```python
from build123d import *

# Parameters (mm, degrees)
BOSS_EXTRUDE1_DEPTH = 3


with BuildPart() as part:
    # Sketch2 → Boss-Extrude1 (new body)
    with BuildSketch(Plane.XY):
        with BuildLine():
            Line((-3.781717443, 11.388529895), (-2.521144962, 7.592353264))
            ThreePointArc((-2.521144962, 7.592353264), (-1.768998185, 7.801964203), (-1, 7.937253933))
            Line((-1, 7.937253933), (-1, 8.94427191))
            Line((-1, 8.94427191), (-1, 9.949874371))
            Line((-1, 9.949874371), (1, 9.949874371))
            Line((1, 9.949874371), (1, 8.94427191))
            Line((1, 8.94427191), (1, 7.937253933))
            ThreePointArc((1, 7.937253933), (8, 0), (1, -7.937253933))
            Line((1, -7.937253933), (1, -8.94427191))
            Line((1, -8.94427191), (1, -10.050125629))
            Line((1, -10.050125629), (-1, -10.050125629))
            Line((-1, -10.050125629), (-1, -8.94427191))
            Line((-1, -8.94427191), (-1, -7.937253933))
            ThreePointArc((-1, -7.937253933), (-1.768998185, -7.801964203), (-2.521144962, -7.592353264))
            Line((-2.521144962, -7.592353264), (-3.781717443, -11.388529895))
            ThreePointArc((-3.781717443, -11.388529895), (12, 0), (-3.781717443, 11.388529895))
        make_face()
    extrude(amount=BOSS_EXTRUDE1_DEPTH)


solid = part.part
```
Geometry: final body of the model. Coordinates: model frame, mm. A direction names the side the tool comes from. Round coordinates to 2 decimals unless told otherwise and drop trailing zeros. Write each loop counter-clockwise with the first axis right and the second up, starting at its lowest first coordinate (ties: lowest second). Pieces come first, ordered by that corner, then holes. Notation, with made-up numbers: (73, -25) -> (105, -25) arc R18 ccw to (105, -11) -> close; hole circle Ø3 at (43, -15). An arc over 180 degrees is marked (long way). Use CSV: the item, a comma, the result in double quotes. Start each with the question number.
Q1. Section B-B (z = 0.3). Return loops of the section in (x, y), plus the area to 3 significant figures.
Q2. Section A-A (x = 0). Return loops of the section in (y, z), plus the area to 3 significant figures.
Q3. First-contact query: pin 1 Ø0.6 at (x, z) = (-0.5, 1) entering from +Y; pin 2 Ø1.7 at (y, z) = (-8.5, 2) entering from -X; pin 3 Ø1.6 at (y, z) = (8.5, 2) entering from +X; pin 4 Ø8 at (x, y) = (-0.5, -1.5) entering from +Z. Flat tips, straight axial feed; report the tip coordinate or a pass-through.
Q4. Pull-direction query (X, two-part tool) for faces 4 (the face through (8, 3, 0)), 5 (the face through (1, -9, 1)), 6 (the face through (-3.16, 9.52, 1.48)); classes: pulls with the +X half, pulls with the -X half, needs draft (parallel to the pull), parting line crosses it, or undercut.
Q5. Section C-C (y = 0). Return loops of the section in (x, z).
Q6. Reachability of faces 1 (the face through (-3.14, -9.46, 1.48)), 2 (the face through (8, 3, 3)), 3 (the face through (8, 0, 1)) from +Z, -Z, +X, -X, +Y, -Y: full face, straight path, thin tool, end or side. Return the list, or none.
Q7. Line query: L1, parallel to Y at x = 0.5, z = 1.15; L2, parallel to Y at x = 3, z = 2.85; L3, parallel to X at y = 8, z = 0.35. Output: solid intervals per line, ascending.
Q8. Section D-D (x = 4.5). Return loops of the section in (y, z), plus the area to 3 significant figures.
Result sheet:
1,outline,"(-3.78, -11.39) arc R12 ccw (long way) to (-3.78, 11.39) -> (-2.52, 7.59) arc R8 cw to (-1, 7.94) -> (-1, 9.95) -> (1, 9.95) -> (1, 7.94) arc R8 cw to (1, -7.94) -> (1, -10.05) -> (-1, -10.05) -> (-1, -7.94) arc R8 cw to (-2.52, -7.59) -> close"
1,area,"143 mm²"
2,outline,"(-12, 0) -> (-10.05, 0) -> (-10.05, 3) -> (-12, 3) -> close; (9.95, 0) -> (12, 0) -> (12, 3) -> (9.95, 3) -> close"
2,area,"12.0 mm²"
3,pin 1,"y = 12"
3,pin 2,"x = -3.1"
3,pin 3,"x = 9.2"
3,pin 4,"through"
4,face 4,"needs draft"
4,face 5,"undercut"
4,face 6,"pulls with the -X half"
5,outline,"(8, 0) -> (12, 0) -> (12, 3) -> (8, 3) -> close"
6,face 1,"+Z, -Z, -X"
6,face 2,"+Z, +X, -X, +Y, -Y"
6,face 3,"+Z, -Z"
7,L1,"-11.99 to -10.05, 9.95 to 11.99"
7,L2,"-11.62 to -7.42, 7.42 to 11.62"
7,L3,"-2.66 to -1, 1 to 8.94"
8,outline,"(-11.12, 0) -> (-6.61, 0) -> (-6.61, 3) -> (-11.12, 3) -> close; (6.61, 0) -> (11.12, 0) -> (11.12, 3) -> (6.61, 3) -> close"
8,area,"27.1 mm²"
